```python
from build123d import *

# Parameters (mm, degrees)
F0_R     = 1.5
F0_R_2   = 5.125
F1_DEPTH = 3
F2_W     = 20
F2_H     = 6.5
F3_DEPTH = 10.5
F5_DEPTH = 6.5
F6_W     = 16
F6_H     = 4.5
F7_DEPTH = 5.7
F8_W     = 10
F8_H     = 12
F9_DEPTH = 5.2


# Not quite as in the source:
# - a pattern or mirror of a feature is missing from the dataset's text; its kind, count and spacing are read off the source's solid


with BuildPart() as f1:
    # F0 (on Top) → F1 (new body)
    with BuildSketch(Plane.XY):
        Polygon((-46.1, 18.13), (-46.1, 0), (46.1, 0), (46.1, 18.13), (27.6, 18.13), (26.6, 17.13), (21, 17.13), (18, 20.13), (18, 44.4), (14, 44.4), (14, 47), (-14, 47), (-14, 44.4), (-18, 44.4), (-18, 20.13), (-21, 17.13), (-26.6, 17.13), (-27.6, 18.13), align=None)
        with Locations((-15, 10)):
            Circle(F0_R, mode=Mode.SUBTRACT)
        with Locations((15, 10)):
            Circle(F0_R, mode=Mode.SUBTRACT)
        with Locations((0, 36.525)):
            Circle(F0_R_2, mode=Mode.SUBTRACT)
    extrude(amount=F1_DEPTH)

    # F2 (on face) → F3 (join)
    with BuildSketch(Plane(origin=(0, 0, 0), x_dir=(1, 0, 0), z_dir=(0, 0, -1))):
        with Locations((-35.1, -8.75)):
            Rectangle(F2_W, F2_H)
    f3 = extrude(amount=F3_DEPTH)

    # F3_copies: F3 across plane
    add(f3.mirror(Plane(origin=(0, 0, 0), x_dir=(0, 0, 1), z_dir=(1, 0, 0))))

    # F4 (on face) → F5 (join, through all)
    with BuildSketch(Plane(origin=(0, 12, 0), x_dir=(-1, 0, 0), z_dir=(0, 1, 0))):
        Polygon((44.5747535126, -14.25), (44.6, -13.9510641961), (27.7299368373, -12.5263106834), (27.9010679845, -10.5), (27.6, -10.5), (27.4057545459, -12.8), align=None)
    f5 = extrude(amount=-F5_DEPTH)

    # F5_copies: F5 across plane
    add(f5.mirror(Plane(origin=(0, 0, 0), x_dir=(0, 0, 1), z_dir=(1, 0, 0))))

    # F6 (on face) → F7 (join)
    with BuildSketch(Plane(origin=(0, 0, 0), x_dir=(1, 0, 0), z_dir=(0, 0, -1))):
        with Locations((0, -10.25)):
            Rectangle(F6_W, F6_H)
    extrude(amount=F7_DEPTH)

    # F8 (on face) → F9 (join)
    with BuildSketch(Plane(origin=(0, 0, 0), x_dir=(1, 0, 0), z_dir=(0, 0, -1))):
        with Locations((-7, 1.5)):
            Rectangle(F8_W, F8_H)
        with Locations((7, 1.5)):
            Rectangle(F8_W, F8_H)
    extrude(amount=F9_DEPTH)


solid = f1.part
```
Verification items for the finished model (mm, model axes). A direction names the side the tool comes from. Give positions to 0.01 mm unless a question says otherwise; leave off trailing zeros. Order: outer loops, then holes, each group sorted by start corner. A loop starts at its lowest first (then second) coordinate and runs counter-clockwise, first axis right, second up. Notation, with made-up numbers: (14.5, 16.5) -> (43.5, 16.5) arc R25 ccw to (43.5, 29.5) -> close; hole circle Ø7 at (17.25, -32). An arc over 180 degrees is marked (long way). One line per item, written item: value.
(1) Sectioned sample at B-B on x = 15. Record the cut outline in (y, z), then the cut area to 3 significant figures.
Final values:
outline: (0, 0) -> (8.5, 0) -> (8.5, 3) -> (0, 3) -> close; (11.5, 0) -> (44.4, 0) -> (44.4, 3) -> (11.5, 3) -> close
area: 124 mm^2
(2) Draft check along Y on faces 1 (the face through (7, -7.5, -3)), 2 (the face through (0, 8, -3)), 3 (the face through (-45.1, 9, -5)), 4 (the face through (-24, 17.13, 1)). Enter one of: pulls with the +Y half, pulls with the -Y half, needs draft (parallel to the pull), parting line crosses it, or undercut.
Final values:
face 1: pulls with the -Y half
face 2: undercut
face 3: needs draft
face 4: pulls with the +Y half
(3) Scan lines: line 1 along Y through (x, z) = (-15, 1.95); line 2 along Y through (x, z) = (0, 2.4); line 3 along Z through (x, y) = (24.5, 5). Record each from-to range of solid material in increasing order. Write a range as [from, to].
Final values:
line 1: [0, 8.5], [11.5, 44.4]
line 2: [0, 31.4], [41.65, 47]
line 3: [0, 3]
(4) Gauge pin test, flat ends, axial feed: pin 1 (2 mm diameter, centred on y = 10, z = -1.5, fed in from -X); pin 2 (1.3 mm diameter, centred on y = 45.5, z = 2, fed in from +X); pin 3 (0.9 mm diameter, centred on x = 40, z = 2, fed in from +Y). Record the tip position at first contact, or that the pin passes through.
Final values:
pin 1: x = -45.1
pin 2: x = 14
pin 3: y = 18.13
(5) Sectioned sample at D-D on x = -10.5. Record the cut outline in (y, z), then the cut area to 3 significant figures.
Final values:
outline: (-7.5, -5.2) -> (4.5, -5.2) -> (4.5, 0) -> (47, 0) -> (47, 3) -> (0, 3) -> (0, 0) -> (-7.5, 0) -> close
area: 203 mm^2
(6) Tool access check on faces 5 (the face through (-7, -2, -5.2)), 6 (the face through (24, 17.13, 1)), 7 (the face through (2, -1, -3)), 8 (the face through (-36.28, 8.8, -13.25)). Record the directions out of +Z, -Z, +X, -X, +Y, -Y that give a thin tool (end or side, any length) a straight path to the whole face; none if there is none.
Final values:
face 5: -Z, +X, -X, -Y
face 6: +Z, -Z, +Y
face 7: -Z, -Y
face 8: -X, +Y, -Y
(7) Sectioned sample at C-C on z = -3. Record the cut outline in (x, y).
Final values:
outline: (-45.1, 5.5) -> (-25.1, 5.5) -> (-25.1, 12) -> (-45.1, 12) -> close; (-12, -7.5) -> (-2, -7.5) -> (-2, 4.5) -> (-12, 4.5) -> close; (-8, 8) -> (8, 8) -> (8, 12.5) -> (-8, 12.5) -> close; (2, -7.5) -> (12, -7.5) -> (12, 4.5) -> (2, 4.5) -> close; (25.1, 5.5) -> (45.1, 5.5) -> (45.1, 12) -> (25.1, 12) -> close
(8) Sectioned sample at A-A on y = -1. Record the cut outline in (x, z).
Final values:
outline: (-12, -5.2) -> (-2, -5.2) -> (-2, 0) -> (-12, 0) -> close; (2, -5.2) -> (12, -5.2) -> (12, 0) -> (2, 0) -> close
